Work out the finished part from the listing and answer in its coordinate system (mm). Give positions to 0.01 mm unless a question says otherwise; leave off trailing zeros. Loops run counter-clockwise (first coordinate to the right, second up) from the corner with the lowest first, then second, coordinate; pieces in that order, holes last.
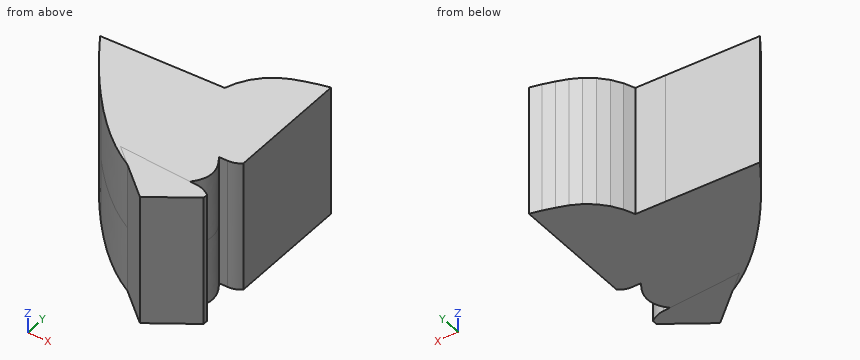
from build123d import *

# Parameters (mm, degrees)
CROQUIS_BASE_DEPTH             = 6.9937
LENTE_PPAL_1_REACH             = 29.176
LENTE_PPAL_1_DIRECTION_2_REACH = 29.176
LENTE_PPAL_2_DEPTH             = 28.175928622
LENTE_PPAL_2_DEPTH_BACK        = 28.175928622
CROQUIS9_3_OUTSIDE_W           = 30.065
CROQUIS9_3_OUTSIDE_H           = 25.937
LENTE_START                    = -6.9937
LENTE_FRONTAL_DEPTH            = 13.9874
LENTE_START_2                  = -6.993701
LENTE_TRASERA_DEPTH            = 13.987402


with BuildPart() as part:
    # Croquis1 → croquis base (new, symmetric)
    with BuildSketch(Plane.XY):
        with BuildLine():
            Line((-8.981845695, 12.608155172), (-23.035921146, 11.871612288))
            Line((-23.035921146, 11.871612288), (-23.035921146, 11.54013782))
            ThreePointArc((-23.035921146, 11.54013782), (-20.949684518, 9.582335705), (-18.945192114, 7.540918896))
            add(Edge.make_bspline(
                [(-18.945192114, 7.540918896), (-10.215008384, -3.697644103), (-2.846604825, -5.059081104)],
                knots=[0.497667241, 0.497667241, 0.497667241, 0.49955428, 0.49955428, 0.49955428], degree=2, weights=[1, 1, 1]))
            add(Edge.make_bspline(
                [(-2.846604825, -5.059081104), (-2.498165198, -4.87297933), (-2.177330418, -4.684462446)],
                knots=[0.498812075, 0.498812075, 0.498812075, 0.498911556, 0.498911556, 0.498911556], degree=2, weights=[1, 1, 1]))
            Line((-2.177330418, -4.684462446), (-2.177330418, 6.186438919))
            add(Edge.make_bspline(
                [(-2.177330418, 6.186438919), (-4.063319702, 8.141636997), (-6.994875026, 10.477389992)],
                knots=[0.50138293, 0.50138293, 0.50138293, 0.502013312, 0.502013312, 0.502013312], degree=2, weights=[1, 1, 1]))
            Line((-6.994875026, 10.477389992), (-8.981845695, 12.608155172))
        make_face()
    extrude(amount=CROQUIS_BASE_DEPTH, both=True)

    # lente ppal 1: up to this face of the body (flat: up to its plane)
    lente_ppal_1_end = Plane(part.part.faces().sort_by_distance((-10.153546236, 5.159655325, 6.9937))[0])
    # Croquis9 → lente ppal 1 (add, up to the picked face)
    with BuildSketch(Plane.XY, mode=Mode.PRIVATE) as lente_ppal_1_sk1:
        with BuildLine():
            add(Edge.make_bspline(
                [(-2.177330418, -4.388282022), (-10.4130765, -4.994158739), (-19.969359014, 9.493765032)],
                knots=[0, 0, 0, 1, 1, 1], degree=2))
            Line((-19.969359014, 9.493765032), (-10.309820395, 10))
            Line((-10.309820395, 10), (-2.177330418, 6.082860828))
            Line((-2.177330418, 6.082860828), (-2.177330418, 2.424232079))
            add(Edge.make_bspline(
                [(-2.177330418, 2.424232079), (-0.304369248, 0.128042884), (-2.177330418, -1.840420572)],
                knots=[0, 0, 0, 1, 1, 1], degree=2))
            Line((-2.177330418, -1.840420572), (-2.177330418, -4.388282022))
        make_face()
    lente_ppal_1_tool1 = split(extrude(lente_ppal_1_sk1.sketch, amount=LENTE_PPAL_1_REACH, mode=Mode.PRIVATE), bisect_by=lente_ppal_1_end, keep=Keep.BOTH, mode=Mode.PRIVATE)
    add(lente_ppal_1_tool1.solids().sort_by(Axis((-9.106368, 3.599172, 0), (0, 0, 1)))[0])

    # lente ppal 1 direction 2: up to this face of the body (flat: up to its plane)
    lente_ppal_1_direction_2_end = Plane(part.part.faces().sort_by_distance((-10.153546236, 5.159655325, -6.9937))[0])
    # Croquis9 → lente ppal 1 direction 2 (add, up to the picked face)
    with BuildSketch(Plane.XY, mode=Mode.PRIVATE) as lente_ppal_1_direction_2_sk1:
        with BuildLine():
            add(Edge.make_bspline(
                [(-2.177330418, -4.388282022), (-10.4130765, -4.994158739), (-19.969359014, 9.493765032)],
                knots=[0, 0, 0, 1, 1, 1], degree=2))
            Line((-19.969359014, 9.493765032), (-10.309820395, 10))
            Line((-10.309820395, 10), (-2.177330418, 6.082860828))
            Line((-2.177330418, 6.082860828), (-2.177330418, 2.424232079))
            add(Edge.make_bspline(
                [(-2.177330418, 2.424232079), (-0.304369248, 0.128042884), (-2.177330418, -1.840420572)],
                knots=[0, 0, 0, 1, 1, 1], degree=2))
            Line((-2.177330418, -1.840420572), (-2.177330418, -4.388282022))
        make_face()
    lente_ppal_1_direction_2_tool1 = split(extrude(lente_ppal_1_direction_2_sk1.sketch, amount=-LENTE_PPAL_1_DIRECTION_2_REACH, mode=Mode.PRIVATE), bisect_by=lente_ppal_1_direction_2_end, keep=Keep.BOTH, mode=Mode.PRIVATE)
    add(lente_ppal_1_direction_2_tool1.solids().sort_by(Axis((-9.106368, 3.599172, 0), (0, 0, -1)))[0])

    # Croquis9<3> outside → lente ppal 2 (cut, two sides: drawn at the far end of the back side and taken through both)
    with BuildSketch(Plane.XY.offset(-LENTE_PPAL_2_DEPTH_BACK)):
        with Locations((-12.1385, 3.7745)):
            Rectangle(CROQUIS9_3_OUTSIDE_W, CROQUIS9_3_OUTSIDE_H)
        with BuildLine():
            Line((-2.177330418, -1.840420572), (-2.177330418, -4.388282022))
            add(Edge.make_bspline(
                [(-2.177330418, -4.388282022), (-10.4130765, -4.994158739), (-19.969359014, 9.493765032)],
                knots=[0, 0, 0, 1, 1, 1], degree=2))
            Line((-19.969359014, 9.493765032), (-10.309820395, 10))
            Line((-10.309820395, 10), (-2.177330418, 6.082860828))
            Line((-2.177330418, 6.082860828), (-2.177330418, 2.424232079))
            add(Edge.make_bspline(
                [(-2.177330418, 2.424232079), (-0.304369248, 0.128042884), (-2.177330418, -1.840420572)],
                knots=[0, 0, 0, 1, 1, 1], degree=2))
        make_face(mode=Mode.SUBTRACT)
    extrude(amount=LENTE_PPAL_2_DEPTH + LENTE_PPAL_2_DEPTH_BACK, mode=Mode.SUBTRACT)

    # Croquis8 → lente frontal (add)
    with BuildSketch(Plane.XY.offset(LENTE_START)):
        with BuildLine():
            Line((0.1, 2.877673418), (0.1, 15.587903347))
            Line((0.1, 15.587903347), (-1.059110992, 15.277320493))
            Line((-1.059110992, 15.277320493), (-2.200378811, 14.9065001))
            Line((-2.200378811, 14.9065001), (-3.324385438, 14.486251242))
            Line((-3.324385438, 14.486251242), (-4.38392255, 13.922885367))
            Line((-4.38392255, 13.922885367), (-5.329535454, 13.184091597))
            Line((-5.329535454, 13.184091597), (-6.132492182, 12.292317806))
            Line((-6.132492182, 12.292317806), (-6.768395299, 11.274660091))
            Line((-6.768395299, 11.274660091), (-7.217923211, 10.162039465))
            Line((-7.217923211, 10.162039465), (-10.309820395, 10))
            Line((-10.309820395, 10), (-2.177330418, 2.342487007))
            Line((-2.177330418, 2.342487007), (-1.190501641, 2.376947827))
            add(Edge.make_bspline(
                [(-1.190501641, 2.376947827), (-0.463368169, 2.402339888), (0.1, 2.877673418)],
                knots=[0, 0, 0, 1, 1, 1], degree=2))
        make_face()
    extrude(amount=LENTE_FRONTAL_DEPTH)

    # Croquis11 → lente trasera (add)
    with BuildSketch(Plane.XY.offset(LENTE_START_2)):
        with BuildLine():
            Line((0.1, -2.367807069), (0.1, -2.867807069))
            Line((0.1, -2.867807069), (-4.373235091, -6))
            Line((-4.373235091, -6), (-9.72117641, -1.512544411))
            Line((-9.72117641, -1.512544411), (-1.458120605, -1.801096678))
            add(Edge.make_bspline(
                [(-1.458120605, -1.801096678), (-0.674591915, -1.828458103), (0.1, -2.367807069)],
                knots=[0, 0, 0, 1, 1, 1], degree=2))
        make_face()
    extrude(amount=LENTE_TRASERA_DEPTH)


solid = part.part
Item 1: Consider line 1 (X direction, y = -4.5, z = -2.25); line 2 (Y direction, x = -12.75, z = -5.5); line 3 (X direction, y = 14, z = 6.25). Determine where each line is inside the solid, lowest interval first.
Item 2: Flat-ended cylindrical pins translate along their axes: pin 1 Ø5 at (x, z) = (-8.5, -2) entering from +Y; pin 2 Ø1.5 at (x, z) = (-5.5, -2.5) entering from +Y; pin 3 Ø1 at (x, z) = (-2, 4.5) entering from -Y. Find the tip coordinate at first contact, or state that the pin passes through.
Item 3: Find section A-A, the plane y = -3.75. Write down the section's boundary in (x, z), plus the area to 3 significant figures.
Ans:
1. line 1: x = -6.16 to -2.23
1. line 2: y = 0.52 to 9.87
1. line 3: x = -4.24 to 0.1
2. pin 1: stops at y = 12.44
2. pin 2: stops at y = 13.64
2. pin 3: stops at y = -4.69
3. outline: (-7.05, -6.99) - (-1.16, -6.99) - (-1.16, 6.99) - (-7.05, 6.99) - close
3. area: 82.5 mm2
